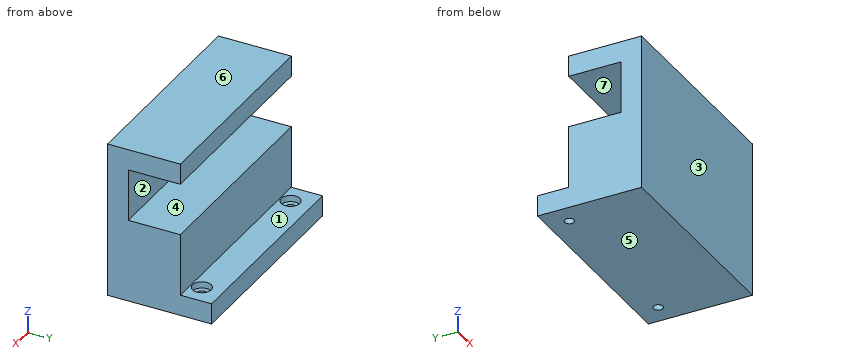
```python
from build123d import *

# Parameters (mm, degrees)
CROQUIS1_W                                           = 100
CROQUIS1_H                                           = 50
SALIENTE_EXTRUIR1_DEPTH                              = 10
CROQUIS2_W                                           = 100
CROQUIS2_H                                           = 10
SALIENTE_EXTRUIR2_DEPTH                              = 75
CROQUIS3_W                                           = 100
CROQUIS3_H                                           = 35
SALIENTE_EXTRUIR3_DEPTH                              = 10
REFRENTADO_PARA_TORNILLO_CON_CABEZA_TRON_D           = 4.5
REFRENTADO_PARA_TORNILLO_CON_CABEZA_TRON_CBORE_D     = 9
REFRENTADO_PARA_TORNILLO_CON_CABEZA_TRON_CBORE_DEPTH = 3.1
CROQUIS11_W                                          = 100
CROQUIS11_H                                          = 35
SALIENTE_EXTRUIR4_DEPTH                              = 30


with BuildPart() as part:
    # Croquis1 → Saliente-Extruir1 (new body)
    with BuildSketch(Plane.XY):
        Rectangle(CROQUIS1_W, CROQUIS1_H)
    extrude(amount=SALIENTE_EXTRUIR1_DEPTH)

    # Croquis2 → Saliente-Extruir2 (add)
    with BuildSketch(Plane.XY):
        with Locations((0, -20)):
            Rectangle(CROQUIS2_W, CROQUIS2_H)
    extrude(amount=SALIENTE_EXTRUIR2_DEPTH)

    # Croquis3 → Saliente-Extruir3 (add)
    with BuildSketch(Plane.XY.offset(75)):
        with Locations((0, -7.5)):
            Rectangle(CROQUIS3_W, CROQUIS3_H)
    extrude(amount=-SALIENTE_EXTRUIR3_DEPTH)

    # Refrentado para tornillo con cabeza troncocónica de M43 (through all)
    with Locations(Plane(origin=(-40, 15, 10), x_dir=(1, 0, 0), z_dir=(0, 0, 1))):
        with Locations((0, 0), (80, 0)):
            CounterBoreHole(REFRENTADO_PARA_TORNILLO_CON_CABEZA_TRON_D / 2, REFRENTADO_PARA_TORNILLO_CON_CABEZA_TRON_CBORE_D / 2, REFRENTADO_PARA_TORNILLO_CON_CABEZA_TRON_CBORE_DEPTH)

    # Croquis11 → Saliente-Extruir4 (add)
    with BuildSketch(Plane.XY.offset(10)):
        with Locations((0, -7.5)):
            Rectangle(CROQUIS11_W, CROQUIS11_H)
    extrude(amount=SALIENTE_EXTRUIR4_DEPTH)


solid = part.part
```
Geometry check sheet. Reference: the model listing, model coordinates, mm. Face numbers are marked on the shaded views. A direction names the side the tool comes from. Give positions to 0.01 mm unless a question says otherwise; leave off trailing zeros. Order: outer loops, then holes, each group sorted by start corner. A loop starts at its lowest first (then second) coordinate and runs counter-clockwise, first axis right, second up. Notation, with made-up numbers: (-32, 58) - (4, 58) arc R18 ccw to (4, 62) - close; hole circle Ø1 at (9.25, -20). An arc over 180 degrees is marked (long way). Answer in a Markdown table with one row per item. Add a question column.
Q1. Material ranges on probe 1 along Z at (x, y) = (17, 5); probe 2 along Y at (x, z) = (-40, 8); probe 3 along Y at (x, z) = (-40, 2.75), recorded low to high. Write a range as from..to.
Q2. Tool access check on the marked faces 1, 2 and 3. Record the directions out of +Z, -Z, +X, -X, +Y, -Y that give a thin tool (end or side, any length) a straight path to the whole face; none if there is none.
Q3. Cross-section at C-C, the plane y = -10.5. Enter the section's corners in (x, z).
Q4. Gauge pin test, flat ends, axial feed: pin 1 (4.5 mm diameter, centred on x = -39, y = 16, fed in from +Z); pin 2 (15 mm diameter, centred on x = 17, z = 30, fed in from +Y); pin 3 (4.5 mm diameter, centred on x = -11.5, y = 16, fed in from +Z). Record the tip position at first contact, or that the pin passes through.
Q5. Mould release check, pull along Z, two halves, no side actions. Record for the marked faces 4, 5, 6 and 7: pulls with the +Z half, pulls with the -Z half, needs draft (parallel to the pull), parting line crosses it, or undercut.
Q6. Cross-section at A-A, the plane y = 15. Enter the section's corners in (x, z).
Q7. Cross-section at B-B, the plane x = 40. Enter the section's corners in (y, z), then the cut area to 3 significant figures.
Q8. Cross-section at D-D, the plane x = -10. Enter the section's corners in (y, z), then the cut area to 3 significant figures.
Check values:
| question | item | result |
|---|---|---|
| 1 | probe 1 | z = 0..40, 65..75 |
| 1 | probe 2 | y = -25..10.5, 19.5..25 |
| 1 | probe 3 | y = -25..12.75, 17.25..25 |
| 2 | face 1 | +Z, +X, -X, +Y |
| 2 | face 2 | +X, -X, +Y |
| 2 | face 3 | +Z, -Z, +X, -X, -Y |
| 3 | outline | (-50, 0) - (50, 0) - (50, 40) - (-50, 40) - close; (-50, 65) - (50, 65) - (50, 75) - (-50, 75) - close |
| 4 | pin 1 | stops at z = 6.9 |
| 4 | pin 2 | stops at y = 10 |
| 4 | pin 3 | stops at z = 10 |
| 5 | face 4 | undercut |
| 5 | face 5 | pulls with the -Z half |
| 5 | face 6 | pulls with the +Z half |
| 5 | face 7 | undercut |
| 6 | outline | (-50, 0) - (-42.25, 0) - (-42.25, 6.9) - (-44.5, 6.9) - (-44.5, 10) - (-50, 10) - close; (-37.75, 0) - (37.75, 0) - (37.75, 6.9) - (35.5, 6.9) - (35.5, 10) - (-35.5, 10) - (-35.5, 6.9) - (-37.75, 6.9) - close; (42.25, 0) - (50, 0) - (50, 10) - (44.5, 10) - (44.5, 6.9) - (42.25, 6.9) - close |
| 7 | outline | (-25, 0) - (12.75, 0) - (12.75, 6.9) - (10.5, 6.9) - (10.5, 10) - (10, 10) - (10, 40) - (-15, 40) - (-15, 65) - (10, 65) - (10, 75) - (-25, 75) - close; (17.25, 0) - (25, 0) - (25, 10) - (19.5, 10) - (19.5, 6.9) - (17.25, 6.9) - close |
| 7 | area | 2,090 mm^2 |
| 8 | outline | (-25, 0) - (25, 0) - (25, 10) - (10, 10) - (10, 40) - (-15, 40) - (-15, 65) - (10, 65) - (10, 75) - (-25, 75) - close |
| 8 | area | 2,150 mm^2 |
